from build123d import *

# Parameters (mm, degrees)
SKETCH1_R             = 12.0777
BOSS_EXTRUDE1_DEPTH   = 3.048
SKETCH2_R             = 9.525
BOSS_EXTRUDE2_DEPTH   = 40
SKETCH3_R             = 9.525
BOSS_EXTRUDE3_DEPTH   = 76.2
M6_TAPPED_HOLE1_D     = 5
M6_TAPPED_HOLE1_DEPTH = 14.986
M6_TAPPED_HOLE1_TIP   = 1.502151548
BOSS_EXTRUDE4_DEPTH   = 4.7625


with BuildPart() as part:
    # Sketch1 → Boss-Extrude1 (new body)
    with BuildSketch(Plane(origin=(0, 0, 0), x_dir=(0, 0, -1), z_dir=(1, 0, 0))):
        Circle(SKETCH1_R)
    extrude(amount=-BOSS_EXTRUDE1_DEPTH)

    # Sketch2 → Boss-Extrude2 (add)
    with BuildSketch(Plane.ZY.offset(3.048)):
        Circle(SKETCH2_R)
    extrude(amount=BOSS_EXTRUDE2_DEPTH)

    # Sketch3 → Boss-Extrude3 (add)
    with BuildSketch(Plane(origin=(0, 0, 0), x_dir=(0, 0, -1), z_dir=(1, 0, 0))):
        Circle(SKETCH3_R)
    extrude(amount=BOSS_EXTRUDE3_DEPTH)

    # M6 Tapped Hole1
    with Locations(Plane(origin=(76.2, 0, 0), x_dir=(0, 0, -1), z_dir=(1, 0, 0))):
        with Locations((0, 0)):
            Hole(M6_TAPPED_HOLE1_D / 2, depth=M6_TAPPED_HOLE1_DEPTH)
            with Locations((0, 0, -(M6_TAPPED_HOLE1_DEPTH + M6_TAPPED_HOLE1_TIP / 2))):  # 118° drill point
                Cone(0, M6_TAPPED_HOLE1_D / 2, M6_TAPPED_HOLE1_TIP, mode=Mode.SUBTRACT)

    # Sketch33 → Boss-Extrude4 (add)
    with BuildSketch(Plane(origin=(0, 6.7818, 0), x_dir=(1, 0, 0), z_dir=(0, 1, 0))):
        with BuildLine():
            Line((12.7, 2.38125), (57.15, 2.38125))
            ThreePointArc((57.15, 2.38125), (59.53125, 0), (57.15, -2.38125))
            Line((57.15, -2.38125), (12.7, -2.38125))
            ThreePointArc((12.7, -2.38125), (10.31875, 0), (12.7, 2.38125))
        make_face()
        with BuildLine():
            Line((-43.048, 2.38125), (-11.298, 2.38125))
            ThreePointArc((-11.298, 2.38125), (-8.91675, 0), (-11.298, -2.38125))
            Line((-11.298, -2.38125), (-43.048, -2.38125))
            Line((-43.048, -2.38125), (-43.048, 2.38125))
        make_face()
    extrude(amount=BOSS_EXTRUDE4_DEPTH)


solid = part.part
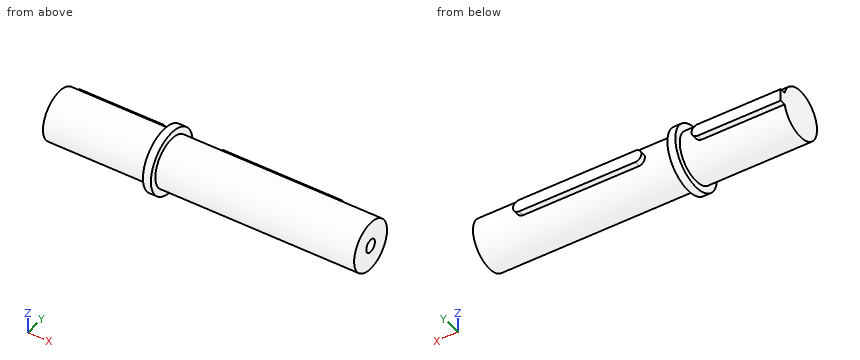
Read the model definition and answer for the solid it produces. Units are mm, in the model's axes. Coordinates: 2 decimals unless noted, no trailing zeros. Loops run counter-clockwise (first coordinate to the right, second up) from the corner with the lowest first, then second, coordinate; pieces in that order, holes last. Notation, with made-up numbers: (34.5, -36) - (93.5, -36) arc R12 ccw to (93.5, -21) - close; hole circle Ø10 at (27, -40). An arc over 180 degrees is marked (long way). Answer in a Markdown table with one row per item.
Q1. Find section B-B on z = -7.75. Write down the section's boundary in (x, y).
Here are the results:
| item | result |
|---|---|
| outline | (-43.05, -5.54) - (-3.05, -5.54) - (-3.05, -9.26) - (0, -9.26) - (0, -5.54) - (76.2, -5.54) - (76.2, 5.54) - (0, 5.54) - (0, 9.26) - (-3.05, 9.26) - (-3.05, 5.54) - (-43.05, 5.54) - close |
Q2. Straight lines are drawn through the part: line 1 along Y through (x, z) = (71.25, 0) (3 decimals); line 2 along Z through (x, y) = (-20, 9.25); line 3 along X through (y, z) = (-4.75, 10.5). For each, find the intervals that lie inside material, in ascending order. Write a range as [from, to].
Here are the results:
| item | result |
|---|---|
| line 1 | y = [-9.525, -2.5], [2.5, 9.525] |
| line 2 | z = [-2.38, 2.38] |
| line 3 | x = [-3.05, 0] |
Q3. Find section A-A on x = 16. Write down the section's boundary in (y, z) (3 decimals), plus the area to 3 significant figures.
Here are the results:
| item | result |
|---|---|
| outline | (9.223, -2.381) - (11.544, -2.381) - (11.544, 2.381) - (9.223, 2.381) arc R9.525 ccw (long way) to start |
| area | 295 mm^2 |
Q4. Find section C-C on y = 7. Write down the section's boundary in (x, z), plus the area to 3 significant figures.
Here are the results:
| item | result |
|---|---|
| outline | (-43.05, -6.46) - (-3.05, -6.46) - (-3.05, -9.84) - (0, -9.84) - (0, -6.46) - (76.2, -6.46) - (76.2, 6.46) - (0, 6.46) - (0, 9.84) - (-3.05, 9.84) - (-3.05, 6.46) - (-43.05, 6.46) - close |
| area | 1,560 mm^2 |
Q5. Given P1, Ø0.7, axis at x = -22, y = 10, coming from the +Z side; P2, Ø10, axis at x = 64, z = 1.5, coming from the -Y side (3 decimals); P3, Ø10, axis at x = -27, y = -3, coming from the +Z side (3 decimals), each flat-ended and moving along its own axis, determine where each tip first touches the part or whether it passes through.
Here are the results:
| item | result |
|---|---|
| P1 | stops at z = 2.38 |
| P2 | stops at y = -9.525 |
| P3 | stops at z = 9.525 |
